For this review, take the finished solid that the model builds, in its own axes (mm). A direction names the side the tool comes from. Give positions to 0.01 mm unless a question says otherwise; leave off trailing zeros. Order: outer loops, then holes, each group sorted by start corner. A loop starts at its lowest first (then second) coordinate and runs counter-clockwise, first axis right, second up.
Item 1: Machinability: for faces 4 (the cylindrical face through (-1.71, 0.12, -0.38)), 5 (the flat face through (0, 9.75, 0)), which of the approach directions +Z, -Z, +X, -X, +Y, -Y give a long, thin tool a straight path to every point of the face, cutting with its end or side? Answer none if there is none.
Item 2: For probe 1 along Y at (x, z) = (-2, -1); probe 2 along X at (y, z) = (-7.75, 0), list the stretches that pass through material, from the lowest coordinate up.
Item 3: Consider section C-C (y = -0.5). Give the boundary of the cut face in (x, z).
Item 4: For P1, Ø2, axis at y = 5.5, z = -2, coming from the -X side; P2, Ø1, axis at x = 0, y = -5, coming from the +Z side, all flat-tipped, find the tip position at first contact; note any pin that passes through.
Item 5: Consider section A-A (x = 0). Give the boundary of the cut face in (y, z).
Item 6: The part is to be moulded in two halves that separate along Y. For faces 1 (the flat face through (2, 8.25, 0)), 2 (the cylindrical face through (-0.9, -9.01, 2.86)), 3 (the flat face through (0, -9.75, 0)), say which applies: released by +Y, released by -Y, zero draft, split by the parting line, or undercut.
Item 7: Consider section B-B (z = 0). Give the boundary of the cut face in (x, y).
```python
from build123d import *

# Parameters (mm, degrees)
SKETCH1_R           = 1.75
BOSS_EXTRUDE1_DEPTH = 8.25


with BuildPart() as part:
    # Sketch1 → Boss-Extrude1 (new, symmetric)
    with BuildSketch(Plane(origin=(0, 0, 0), x_dir=(1, 0, 0), z_dir=(0, 1, 0))):
        with Locations(Location((0, 0, 0), (0, 0, 270))):
            Circle(SKETCH1_R)
    extrude(amount=BOSS_EXTRUDE1_DEPTH, both=True)

    # Sketch2 → Revolve2 (revolve)
    with BuildSketch(Plane.XY, mode=Mode.PRIVATE) as revolve2_sk:
        with BuildLine():
            Line((-2.8, 8.25), (0, 8.25))
            Line((0, 8.25), (0, 9.75))
            Line((0, 9.75), (-2.8, 9.75))
            ThreePointArc((-2.8, 9.75), (-2.941421356, 9.691421356), (-3, 9.55))
            Line((-3, 9.55), (-3, 8.45))
            ThreePointArc((-3, 8.45), (-2.941421356, 8.308578644), (-2.8, 8.25))
        make_face()
        with BuildLine():
            Line((0, -9.75), (0, -8.25))
            Line((0, -8.25), (-2.8, -8.25))
            ThreePointArc((-2.8, -8.25), (-2.941421356, -8.308578644), (-3, -8.45))
            Line((-3, -8.45), (-3, -9.55))
            ThreePointArc((-3, -9.55), (-2.941421356, -9.691421356), (-2.8, -9.75))
            Line((-2.8, -9.75), (0, -9.75))
        make_face()
    revolve(revolve2_sk.sketch.rotate(Axis((0, 9.75, 0), (0, -1, 0)), 270), axis=Axis((0, 9.75, 0), (0, -1, 0)))


solid = part.part
```
Resolved:
1. face 4: none
1. face 5: +Z, -Z, +X, -X, +Y
2. probe 1: y = -9.75 to -8.25, 8.25 to 9.75
2. probe 2: x = -1.75 to 1.75
3. outline: circle Ø3.5 at (0, 0)
4. P1: stops at x = -1.44
4. P2: stops at z = 1.75
5. outline: (-9.75, -2.8) arc R0.2 ccw to (-9.55, -3) - (-8.45, -3) arc R0.2 ccw to (-8.25, -2.8) - (-8.25, -1.75) - (8.25, -1.75) - (8.25, -2.8) arc R0.2 ccw to (8.45, -3) - (9.55, -3) arc R0.2 ccw to (9.75, -2.8) - (9.75, 2.8) arc R0.2 ccw to (9.55, 3) - (8.45, 3) arc R0.2 ccw to (8.25, 2.8) - (8.25, 1.75) - (-8.25, 1.75) - (-8.25, 2.8) arc R0.2 ccw to (-8.45, 3) - (-9.55, 3) arc R0.2 ccw to (-9.75, 2.8) - close
6. face 1: undercut
6. face 2: zero draft
6. face 3: released by -Y
7. outline: (-3, -9.55) arc R0.2 ccw to (-2.8, -9.75) - (2.8, -9.75) arc R0.2 ccw to (3, -9.55) - (3, -8.45) arc R0.2 ccw to (2.8, -8.25) - (1.75, -8.25) - (1.75, 8.25) - (2.8, 8.25) arc R0.2 ccw to (3, 8.45) - (3, 9.55) arc R0.2 ccw to (2.8, 9.75) - (-2.8, 9.75) arc R0.2 ccw to (-3, 9.55) - (-3, 8.45) arc R0.2 ccw to (-2.8, 8.25) - (-1.75, 8.25) - (-1.75, -8.25) - (-2.8, -8.25) arc R0.2 ccw to (-3, -8.45) - close
